```python
from build123d import *

# Parameters (mm, degrees)
BOSS_EXTRUDE1_DEPTH = 15
FILLET1_R           = 20
CUT_EXTRUDE1_START  = -15
CUT_EXTRUDE1_DEPTH  = 15
BOSS_EXTRUDE2_START = -15
BOSS_EXTRUDE2_DEPTH = 15


with BuildPart() as part:
    # Sketch1 → Boss-Extrude1 (new body)
    # profile 1 of 6: a face of its own
    with BuildSketch(Plane.XY):
        with BuildLine():
            Line((-20, -30), (-30, -30))
            ThreePointArc((-30, -30), (-29.388396861, -36.026784376), (-27.578524672, -41.807835403))
            Line((-27.578524672, -41.807835403), (-20, -30))
        make_face()
    # profile 2 of 6: a face of its own
    with BuildSketch(Plane.XY):
        with BuildLine():
            Line((0, -10), (0, 0))
            ThreePointArc((0, 0), (-21.213203436, -8.786796564), (-30, -30))
            Line((-30, -30), (-20, -30))
            ThreePointArc((-20, -30), (-14.142135624, -15.857864376), (0, -10))
        make_face()
    # profile 3 of 6: a face of its own
    with BuildSketch(Plane.XY):
        with BuildLine():
            Line((0, -60), (0, -50))
            ThreePointArc((0, -50), (-14.142135624, -44.142135624), (-20, -30))
            Line((-20, -30), (-27.578524672, -41.807835403))
            ThreePointArc((-27.578524672, -41.807835403), (-16.519154608, -55.04231481), (0, -60))
        make_face()
    # profile 4 of 6: a face of its own
    with BuildSketch(Plane.XY):
        with BuildLine():
            ThreePointArc((-27.578524672, -41.807835403), (-29.388396861, -36.026784376), (-30, -30))
            Line((-30, -30), (-49.254650189, -60))
            Line((-49.254650189, -60), (-30, -105))
            ThreePointArc((-30, -105), (-28.650020621, -98.780921528), (-24.84307506, -93.681260081))
            Line((-24.84307506, -93.681260081), (-39.254650189, -60))
            Line((-39.254650189, -60), (-27.578524672, -41.807835403))
        make_face()
    # profile 5 of 6: a face of its own
    with BuildSketch(Plane.XY):
        with BuildLine():
            ThreePointArc((-24.84307506, -93.681260081), (-28.650020621, -98.780921528), (-30, -105))
            Line((-30, -105), (-20, -105))
            Line((-20, -105), (-24.84307506, -93.681260081))
        make_face()
    # profile 6 of 6: a face of its own
    with BuildSketch(Plane.XY):
        with BuildLine():
            Line((-20, -105), (-30, -105))
            ThreePointArc((-30, -105), (-15, -120), (0, -105))
            ThreePointArc((0, -105), (-8.780921528, -91.349979379), (-24.84307506, -93.681260081))
            Line((-24.84307506, -93.681260081), (-20, -105))
        make_face()
        with BuildLine():
            ThreePointArc((-10, -105), (-15, -110), (-20, -105))
            ThreePointArc((-20, -105), (-15, -100), (-10, -105))
        make_face(mode=Mode.SUBTRACT)
    extrude(amount=BOSS_EXTRUDE1_DEPTH)

    # Fillet1
    fillet1_edges = [part.edges().sort_by_distance(p)[0] for p in [
        (-39.254650189, -60, 7.5),
        (-49.254650189, -60, 7.5),
    ]]
    fillet(fillet1_edges, radius=FILLET1_R)

    # Sketch2 → Cut-Extrude1 (cut)
    with BuildSketch(Plane.XY.offset(15).offset(CUT_EXTRUDE1_START)):
        with BuildLine():
            Line((-15, -90), (-15, -92.5))
            ThreePointArc((-15, -92.5), (-3.506810704, -109.914936399), (-24.038127106, -113.634944031))
            Line((-24.038127106, -113.634944031), (-25.845752528, -115.361932837))
            ThreePointArc((-25.845752528, -115.361932837), (-1.208172845, -110.897923679), (-15, -90))
        make_face()
    extrude(amount=CUT_EXTRUDE1_DEPTH, mode=Mode.SUBTRACT)

    # Sketch3 → Boss-Extrude2 (add)
    with BuildSketch(Plane.XY.offset(15).offset(BOSS_EXTRUDE2_START)):
        with BuildLine():
            Line((-14.5, -90), (-15, -90))
            Line((-15, -90), (-15, -92.5))
            ThreePointArc((-15, -92.5), (-14.279138, -92.520802992), (-13.560675373, -92.583142724))
            Line((-13.560675373, -92.583142724), (-14.5, -90))
        make_face()
        with BuildLine():
            Line((-10.840273343, -90.579643758), (-12.53185915, -92.746091205))
            ThreePointArc((-12.53185915, -92.746091205), (-11.13728757, -93.111793546), (-9.79410102, -93.635642746))
            Line((-9.79410102, -93.635642746), (-9.889216826, -90.888660753))
            Line((-9.889216826, -90.888660753), (-10.840273343, -90.579643758))
        make_face()
        with BuildLine():
            Line((-6.587729713, -92.570852458), (-8.865992497, -94.108537658))
            ThreePointArc((-8.865992497, -94.108537658), (-7.652684346, -94.88728757), (-6.53711633, -95.800565236))
            Line((-6.53711633, -95.800565236), (-5.778712718, -93.158637711))
            Line((-5.778712718, -93.158637711), (-6.587729713, -92.570852458))
        make_face()
        with BuildLine():
            Line((-3.158637711, -95.778712718), (-5.800565236, -96.53711633))
            ThreePointArc((-5.800565236, -96.53711633), (-4.88728757, -97.652684346), (-4.108537658, -98.865992497))
            Line((-4.108537658, -98.865992497), (-2.570852458, -96.587729713))
            Line((-2.570852458, -96.587729713), (-3.158637711, -95.778712718))
        make_face()
        with BuildLine():
            Line((-0.888660753, -99.889216826), (-3.635642746, -99.79410102))
            ThreePointArc((-3.635642746, -99.79410102), (-3.111793546, -101.13728757), (-2.746091205, -102.53185915))
            Line((-2.746091205, -102.53185915), (-0.579643758, -100.840273343))
            Line((-0.579643758, -100.840273343), (-0.888660753, -99.889216826))
        make_face()
        with BuildLine():
            Line((0, -104.5), (-2.583142724, -103.560675373))
            ThreePointArc((-2.583142724, -103.560675373), (-2.5, -105), (-2.583142724, -106.439324627))
            Line((-2.583142724, -106.439324627), (0, -105.5))
            Line((0, -105.5), (0, -104.5))
        make_face()
        with BuildLine():
            Line((-0.579643758, -109.159726657), (-2.746091205, -107.46814085))
            ThreePointArc((-2.746091205, -107.46814085), (-3.111793546, -108.86271243), (-3.635642746, -110.20589898))
            Line((-3.635642746, -110.20589898), (-0.888660753, -110.110783174))
            Line((-0.888660753, -110.110783174), (-0.579643758, -109.159726657))
        make_face()
        with BuildLine():
            ThreePointArc((-21.134007503, -115.891462342), (-22.347315654, -115.11271243), (-23.46288367, -114.199434764))
            Line((-23.46288367, -114.199434764), (-24.221287282, -116.841362289))
            Line((-24.221287282, -116.841362289), (-23.412270287, -117.429147542))
            Line((-23.412270287, -117.429147542), (-21.134007503, -115.891462342))
        make_face()
        with BuildLine():
            Line((-2.570852458, -113.412270287), (-4.108537658, -111.134007503))
            ThreePointArc((-4.108537658, -111.134007503), (-4.88728757, -112.347315654), (-5.800565236, -113.46288367))
            Line((-5.800565236, -113.46288367), (-3.158637711, -114.221287282))
            Line((-3.158637711, -114.221287282), (-2.570852458, -113.412270287))
        make_face()
        with BuildLine():
            ThreePointArc((-17.46814085, -117.253908795), (-18.86271243, -116.888206454), (-20.20589898, -116.364357254))
            Line((-20.20589898, -116.364357254), (-20.110783174, -119.111339247))
            Line((-20.110783174, -119.111339247), (-19.159726657, -119.420356242))
            Line((-19.159726657, -119.420356242), (-17.46814085, -117.253908795))
        make_face()
        with BuildLine():
            Line((-5.778712718, -116.841362289), (-6.53711633, -114.199434764))
            ThreePointArc((-6.53711633, -114.199434764), (-7.652684346, -115.11271243), (-8.865992497, -115.891462342))
            Line((-8.865992497, -115.891462342), (-6.587729713, -117.429147542))
            Line((-6.587729713, -117.429147542), (-5.778712718, -116.841362289))
        make_face()
        with BuildLine():
            ThreePointArc((-13.560675373, -117.416857276), (-15, -117.5), (-16.439324627, -117.416857276))
            Line((-16.439324627, -117.416857276), (-15.5, -120))
            Line((-15.5, -120), (-14.5, -120))
            Line((-14.5, -120), (-13.560675373, -117.416857276))
        make_face()
        with BuildLine():
            Line((-9.889216826, -119.111339247), (-9.79410102, -116.364357254))
            ThreePointArc((-9.79410102, -116.364357254), (-11.13728757, -116.888206454), (-12.53185915, -117.253908795))
            Line((-12.53185915, -117.253908795), (-10.840273343, -119.420356242))
            Line((-10.840273343, -119.420356242), (-9.889216826, -119.111339247))
        make_face()
    extrude(amount=BOSS_EXTRUDE2_DEPTH)


solid = part.part
```
Design review of the part built by this model. Coordinates are the model's own, in mm. A direction names the side the tool comes from. Coordinates: 2 decimals unless noted, no trailing zeros. Order: outer loops, then holes, each group sorted by start corner. A loop starts at its lowest first (then second) coordinate and runs counter-clockwise, first axis right, second up. Notation, with made-up numbers: (-12.75, 12) -> (10.25, 12) arc R11 ccw to (10.25, 17) -> close; hole circle Ø5 at (-22.75, 58). An arc over 180 degrees is marked (long way). One line per item, written item: value. Start each with the question number.
Q1. For probe 1 along X at (y, z) = (-30, 10.75); probe 2 along Y at (x, z) = (-10.5, 8.5); probe 3 along X at (y, z) = (-80, 13.75), list the stretches that pass through material, from the lowest coordinate up.
Q2. Mouldability with a two-part tool opening along X and no side actions: class faces 6 (the flat face through (-13, -55, 0)), 7 (the flat face through (-7.74, -116.65, 7.4)), 8 (the cylindrical face through (-46.64, -60.36, 7.6)), 9 (the flat face through (-1.31, -105.976, 7.395)) as pulls with the +X half, pulls with the -X half, needs draft (parallel to the pull), parting line crosses it, or undercut.
Q3. Take a section at A-A, the plane y = -83.5. State the section outline as (x, z) points.
Q4. Tool access review of faces 1 (the flat face through (-11.674, -91.648, 7.395)), 2 (the flat face through (-1.27, -104.04, 7.4)), 3 (the cylindrical face through (-20.979, -8.555, 7.395)), 4 (the flat face through (-18.326, -118.352, 7.395)), 5 (the flat face through (0, -55, 7)): name each direction out of +Z, -Z, +X, -X, +Y, -Y from which nothing blocks a thin tool from reaching the whole face with its end or side.
Q5. Insertion check: pin 1 Ø2 at (x, z) = (-22.5, 8.5) entering from +Y; pin 2 Ø8 at (x, z) = (-9.5, 2) entering from +Y; pin 3 Ø1.5 at (x, z) = (-37, 5.5) entering from -Y; pin 4 Ø1 at (x, y) = (-38.5, -57.5) entering from -Z. Each pin has a flat end and moves straight along its axis. Give the tip position at first contact, or say it passes through.
Q6. Take a section at B-B, the plane y = -17.5. State the section outline as (x, z) points.
Values follow:
1. probe 1: x = -30 to -20
1. probe 2: y = -119.31 to -107.18, -102.82 to -90.69, -58.1 to -47.02, -12.98 to -1.9
1. probe 3: x = -40.7 to -30.7
2. face 6: needs draft
2. face 7: undercut
2. face 8: pulls with the -X half
2. face 9: pulls with the +X half
3. outline: (-39.2, 0) -> (-29.2, 0) -> (-29.2, 15) -> (-39.2, 15) -> close
4. face 1: +Z, -Z
4. face 2: +Z, -Z, +X
4. face 3: +Z, -Z, -X, +Y
4. face 4: +Z, -Z, -Y
4. face 5: +Z, -Z, +X, +Y, -Y
5. pin 1: stops at y = -9.08
5. pin 2: stops at y = -0.51
5. pin 3: stops at y = -90.39
5. pin 4: stops at z = 0
6. outline: (-27.27, 0) -> (-15.61, 0) -> (-15.61, 15) -> (-27.27, 15) -> close
